Model file for the job. Use its own axes, mm. Face numbers are marked on the shaded views. A direction names the side the tool comes from. Coordinates: 2 decimals unless noted, no trailing zeros. Write each loop counter-clockwise with the first axis right and the second up, starting at its lowest first coordinate (ties: lowest second). Pieces come first, ordered by that corner, then holes. Notation, with made-up numbers: (81, 50) -> (90, 50) arc R25 ccw to (90, 87) -> close; hole circle Ø7 at (49.5, -17.75). An arc over 180 degrees is marked (long way). Write item = value, one per line. Start each with the question number.
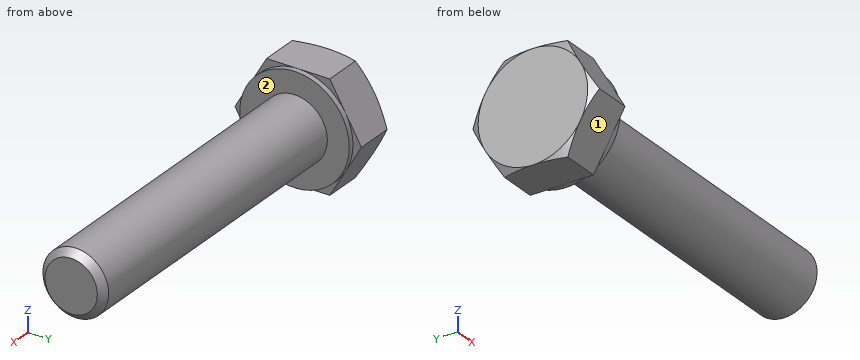
Autodesk Inventor part; units mm, degrees
ref_plane "Work Plane1" through (1.525, 0, 0) normal (0, 0, 1) x (1, 0, 0)
ref_plane "YZ Plane" through (0, 0, 0) normal (1, 0, 0) x (0, 1, 0)
ref_plane "XZ Plane" through (0, 0, 0) normal (0, 1, 0) x (-1, 0, 0)
sketch "Sketch1" plane through (0, 0, 0) normal (0, 0, 1) x (1, 0, 0)
  line L0 (0, 5) -> (0, 3)
  line L1 (12, 3) -> (30, 3)
  line L2 (30, 3) -> (30, 0)
  line L3 (30, 0) -> (-0.5001, 0)
  line L4 (-6.6001, 0) -> (36.1, 0)
  line L5 (-0.5001, 0) -> (-0.5001, 5)
  line L6 (-0.5001, 5) -> (0, 5)
  line L7 (12, 3) -> (11.3865, 3)
  line L8 (11.3865, 3) -> (0, 3)
  line L9 (0, -1) -> (0, 6)
  dimension "d0" = 30
  dimension "d1" = 18
  dimension "d2" = 6
  dimension "d9" = 0.5001
  dimension "d10" = 10
  dimension "d13" = 0.6136
  dimension "d14" = 6
revolve "Body" add sketch "Sketch1" angle 360 about axis through (30, 0, 0) along (-1, 0, 0)
sketch "Sketch2" plane through (-0.5001, 0, 0) normal (-1, 0, 0) x (0, 0, 1)
  line L0 (0, 5.7735) -> (5, 2.8868)
  line L1 (5, 2.8868) -> (5, -2.8868)
  line L2 (5, -2.8868) -> (0, -5.7735)
  line L3 (0, -5.7735) -> (-5, -2.8868)
  line L4 (-5, -2.8868) -> (-5, 2.8868)
  line L5 (-5, 2.8868) -> (0, 5.7735)
  point P0 (0, 0)
  point P1 (0, 0)
  dimension "d11" = 10
extrude "Head" add sketch "Sketch2" along normal blind 3.88
sketch "Sketch4" plane through (0, 0, 0) normal (0, 0, 1) x (1, 0, 0)
  line L0 (-4.3801, 5) -> (-4.3801, 5.7735)
  line L1 (-4.3801, 5.7735) -> (-3.9335, 5.7735)
  line L2 (-3.9335, 5.7735) -> (-4.3801, 5)
  line L3 (-5.1561, 0) -> (0.2759, 0)
  line L4 (-0.5001, 5.7735) -> (-4.3801, 5.7735)
  line L5 (-4.3801, 2.8868) -> (-4.3801, 5.7735)
  dimension "d5" = 30
  dimension "d19" = 10
revolve "Chamfer1" cut sketch "Sketch4" angle 360 about axis through (-10, 0, 0) along (1, 0, 0)
thread "Thread"
chamfer "Chamfer2" distance 0.6135 distance2 0.6136 1 edges at (30, -3, 0) measured on face at (30, 1.1079, -0.4377)
ref_plane "Work Plane1" through (1.525, 0, 0) normal (0, 0, 1) x (1, 0, 0)
equation "\"d11\" = SW"
equation "\"d3\" = KOH - SD"
equation "\"d15\" = GEL"
equation "\"d6\" = -0.5 * SPD + 0.5 * GD"
equation "\"d0\" = NLG"
equation "\"d1\" = GEL"
equation "\"d2\" = GD"
equation "\"d10\" = SD2"
equation "\"d14\" = BDM"
equation "\"d5\" = ANG1"
equation "\"d19\" = SW0"
equation "\"NLG\" = 30"
equation "\"GD\" = NND"
equation "\"BDM\" = NND"
equation "\"KOH\" = 4.38"
equation "\"GEL\" = 18"
equation "\"SW\" = 10"
equation "\"SW0\" = SW"
equation "\"SPD\" = NND - 1.2269 * PTC"
equation "\"SD2\" = SW"
equation "\"SD\" = 0.5"
equation "\"ANG1\" = 30deg"
equation "\"GAL\" = 0.61345 * PTC"
equation "\"GUL\" = 0.61345 * PTC"
equation "\"RR\" = 0.25"
equation "\"WFT\" = SD"
equation "\"GD1\" = THREADDIA - 1.2269 * PTC"
equation "\"THREADDIA\" = 6"
equation "\"TOA\" = 30deg"
equation "\"FAWI\" = 45deg"
equation "\"PTC\" = 1"
equation "\"NND\" = 6"
equation "\"E0\" = 1.155 * SW"
properties part number "AS 1111 - M6 x 30" material "Steel, Mild"
(1) 3-axis set-ups, long thin cutter, end or side, ignore diameter. For the marked faces 1 and 2: which of +Z, -Z, +X, -X, +Y, -Y reach the whole face in a straight line?
(2) Drill centre lines: line 1 along X through (y, z) = (-1.5, -4); line 2 along X through (y, z) = (5, -1); line 3 along Y through (x, z) = (4.5, -0.75). Where is each one in solid material? Low to high.
(3) Saw through at A-A (x = 10.5). Give the cut face in (y, z), then the cut area to 3 significant figures.
(4) Drop flat-ended pins along their axis: pin 1 Ø1.3 at (y, z) = (2, 4) entering from +X; pin 2 Ø0.7 at (y, z) = (5.5, 1) entering from +X; pin 3 Ø1 at (x, y) = (23, 2.5) entering from +Z; pin 4 Ø6 at (y, z) = (-1.5, 2.5) entering from +X. Give the stop position or say it passes through.
Returned:
q1.face_1 = -Z, +X, -X, -Y
q1.face_2 = +X
q2.line_1 = -4.38 to 0
q2.line_2 = -4.32 to -0.5
q2.line_3 = -2.9 to 2.9
q3.outline = circle Ø6 at (0, 0)
q3.area = 28.3 mm2
q4.pin_1 = 0
q4.pin_2 = -0.5
q4.pin_3 = 2.24
q4.pin_4 = 30
